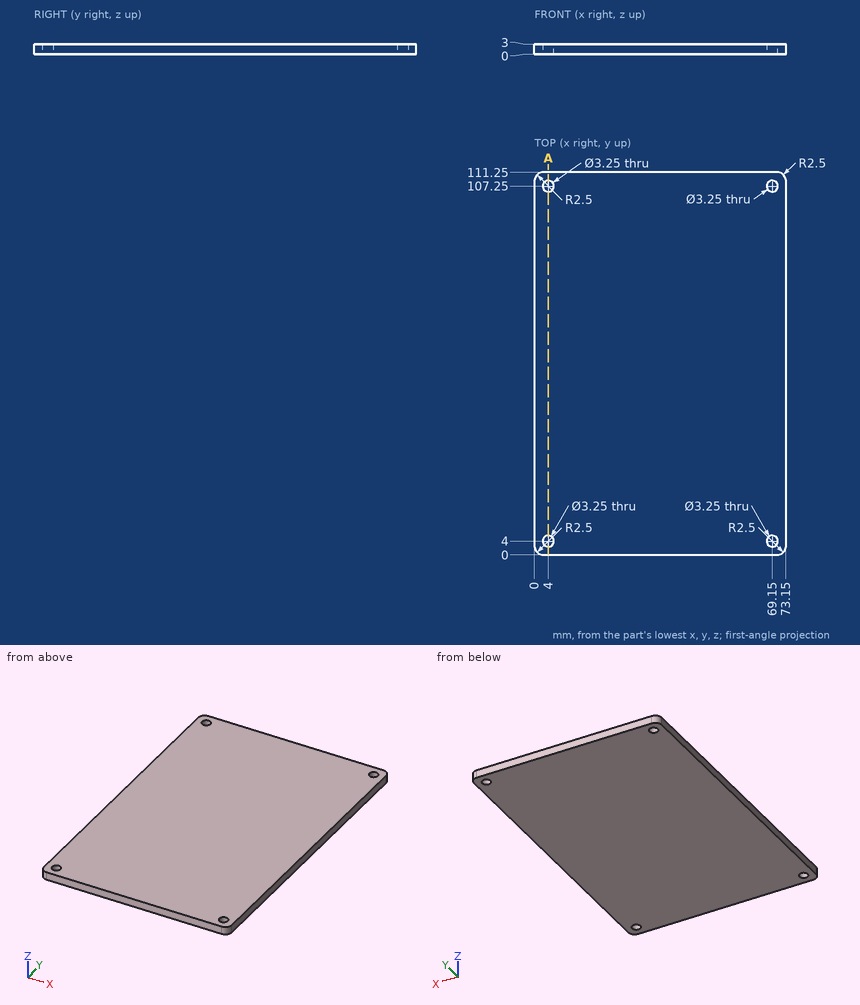
Input: dimensioned drawing with shaded views. Units: mm. Origin: part minimum x, y, z. Round coordinates to 2 decimals unless told otherwise and drop trailing zeros. Return JSON: item names as keys, results as strings. Group by question number.
1. Pin query (flat end, axial travel): pin 1 (2.5 mm diameter, centred on x = 4, y = 4, fed in from -Z). Return the tip coordinate at first contact, or that it passes through.
2. Material intervals for line 1 along Y through (x, z) = (4.5, 2.8); line 2 along Y through (x, z) = (68, 2.4), sorted ascending. Write a range as from..to.
3. Section query A-A on x = 4. State how many separate pieces and enclosed holes the cut face has, and give its area (3 significant figures).
Checks:
{
 "1": {"pin 1": "passes through"},
 "2": {"line 1": "y = 0..2.45, 5.55..105.7, 108.8..111.25", "line 2": "y = 0..2.85, 5.15..106.1, 108.4..111.25"},
 "3": {"separate pieces": "3", "enclosed holes": "0", "area": "314 mm²"}
}
